Part print with two shaded views. Sizes in mm from the minimum x, y, z corner. A direction names the side the tool comes from. Round coordinates to 2 decimals unless told otherwise and drop trailing zeros. Order: outer loops, then holes, each group sorted by start corner. A loop starts at its lowest first (then second) coordinate and runs counter-clockwise, first axis right, second up. Notation, with made-up numbers: (46, -12.75) -> (85, -12.75) arc R22 ccw to (85, 24.25) -> close; hole circle Ø8 at (79, 78.25). An arc over 180 degrees is marked (long way). Use a Markdown table: item, result. Add a question column.
Item 1: Probe L1, parallel to X at y = 15, z = 44; L2, parallel to Y at x = 58, z = 8; L3, parallel to Z at x = 40, y = 24. List the from-to ranges inside material, lowest first.
Item 2: Pin check, flat tips, straight feed: pin 1 (10 mm diameter, centred on y = 41, z = 37, fed in from +X); pin 2 (4 mm diameter, centred on x = 34.5, y = 49, fed in from +Z); pin 3 (1 mm diameter, centred on y = 40, z = 48, fed in from -X). Stop position of each tip, or through.
Item 3: Slice it at B-B, the plane y = 35. Give the cut face in (x, z).
Item 4: 3-axis set-ups, long thin cutter, end or side, ignore diameter. For the marked faces 4, 5, 6 and 7: which of +Z, -Z, +X, -X, +Y, -Y reach the whole face in a straight line?
Item 5: Slice it at D-D, the plane z = 5. Give the cut face in (x, y).
Item 6: Two-plate mould, pull along X, no slides. Class the marked faces 1, 2 and 3: released by +X, released by -X, zero draft, split by the parting line, or undercut.
Item 7: Slice it at A-A, the plane z = 39. Give the cut face in (x, y).
Item 8: Slice it at C-C, the plane x = 68. Give the cut face in (y, z).
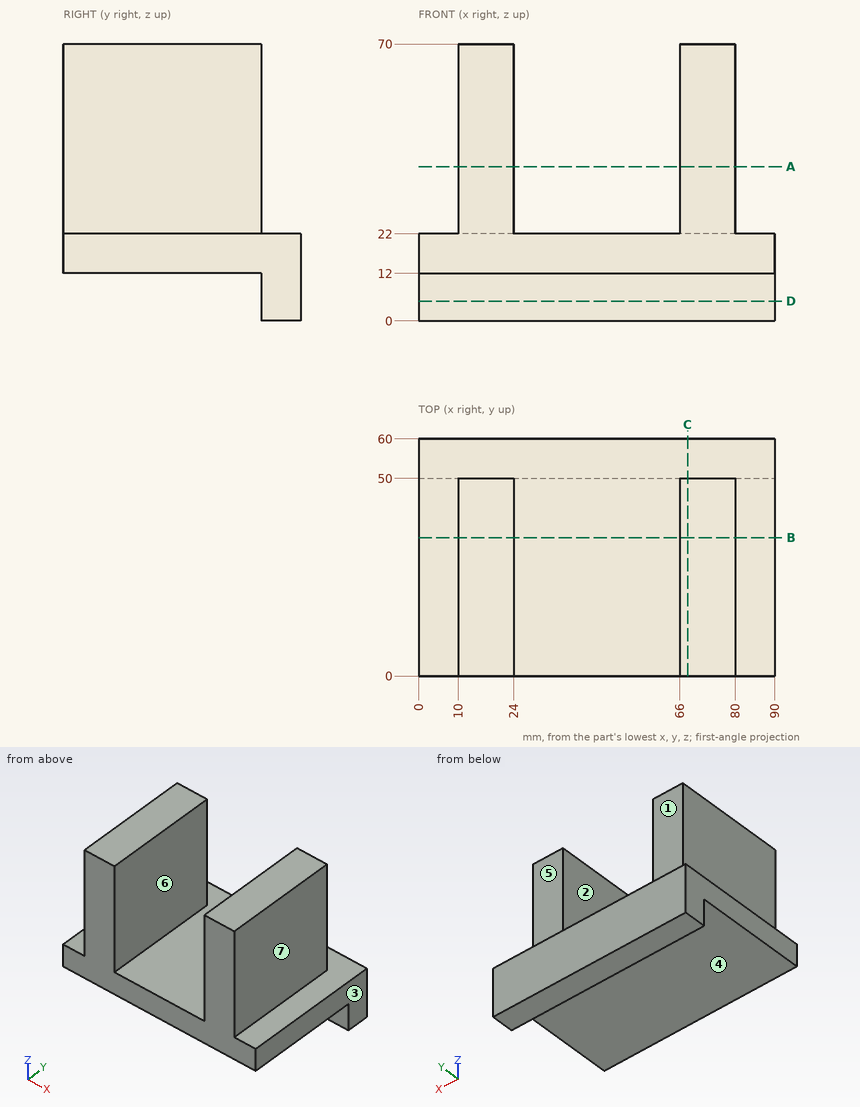
Check sheet entries:
| question | item | result |
|---|---|---|
| 1 | L1 | 10 to 24, 66 to 80 |
| 1 | L2 | 50 to 60 |
| 1 | L3 | 12 to 22 |
| 2 | pin 1 | x = 80 |
| 2 | pin 2 | z = 22 |
| 2 | pin 3 | x = 10 |
| 3 | outline | (0, 12) -> (90, 12) -> (90, 22) -> (80, 22) -> (80, 70) -> (66, 70) -> (66, 22) -> (24, 22) -> (24, 70) -> (10, 70) -> (10, 22) -> (0, 22) -> close |
| 4 | face 4 | -Z, +X, -X, -Y |
| 4 | face 5 | +Z, +X, -X, +Y |
| 4 | face 6 | +Z, +Y, -Y |
| 4 | face 7 | +Z, +X, +Y, -Y |
| 5 | outline | (0, 50) -> (90, 50) -> (90, 60) -> (0, 60) -> close |
| 6 | face 1 | zero draft |
| 6 | face 2 | undercut |
| 6 | face 3 | released by +X |
| 7 | outline | (10, 0) -> (24, 0) -> (24, 50) -> (10, 50) -> close; (66, 0) -> (80, 0) -> (80, 50) -> (66, 50) -> close |
| 8 | outline | (0, 12) -> (50, 12) -> (50, 0) -> (60, 0) -> (60, 22) -> (50, 22) -> (50, 70) -> (0, 70) -> close |
